Design review of the part built by this model. Coordinates are the model's own, in mm. A direction names the side the tool comes from. Give positions to 0.01 mm unless a question says otherwise; leave off trailing zeros. Order: outer loops, then holes, each group sorted by start corner. A loop starts at its lowest first (then second) coordinate and runs counter-clockwise, first axis right, second up. Notation, with made-up numbers: M 57,-8.75 L 78,-8.75 A18 ccw 78,7.25 Z; hole C 71.5,33.5 d4. An arc over 180 degrees is marked long. Answer as a JSON object with one key per item and string values.
from build123d import *

# Parameters (mm, degrees)
CHAMFER1_SIZE      = 2
CUT_EXTRUDE1_DEPTH = 5


with BuildPart() as part:
    # Sketch1 → Revolve1 (revolve)
    with BuildSketch(Plane.XY):
        Polygon((0, 0), (0, 22.5), (65, 22.5), (65, 27), (70, 27), (70, 52), (80, 52), (80, 35), (155, 35), (155, 52), (165, 52), (165, 24.5), (174, 24.5), (174, 21), (234, 21), (234, 0), align=None)
    revolve(axis=Axis((0, 0, 0), (1, 0, 0)))

    # Chamfer1
    chamfer1_edges = [part.edges().sort_by_distance(p)[0] for p in [
        (165, -24.5, 0),
        (155, -35, 0),
        (80, -35, 0),
    ]]
    chamfer(chamfer1_edges, length=CHAMFER1_SIZE)

    # Sketch2 → Cut-Extrude1 (cut)
    with BuildSketch(Plane(origin=(0, 21, 0), x_dir=(1, 0, 0), z_dir=(0, 1, 0))):
        with BuildLine():
            Line((204, 6), (204, -6))
            Line((204, -6), (184, -6))
            ThreePointArc((184, -6), (178, 0), (184, 6))
            Line((184, 6), (204, 6))
        make_face()
    cut_extrude1 = extrude(amount=-CUT_EXTRUDE1_DEPTH, mode=Mode.SUBTRACT)

    # Mirror1: Cut-Extrude1 across plane
    add(cut_extrude1.mirror(Plane(origin=(204, 16, -6), x_dir=(0, 0, 1), z_dir=(1, 0, 0))), mode=Mode.SUBTRACT)


solid = part.part
(1) We need section A-A (z = -44.5). Write out the cut boundary in (x, y).
Checked values:
{"outline": "M 70,-26.9 L 80,-26.9 L 80,26.9 L 70,26.9 Z; M 155,-26.9 L 165,-26.9 L 165,26.9 L 155,26.9 Z"}
(2) To check wall thickness, follow L1, parallel to X at y = 38, z = 28.5; L2, parallel to Z at x = 172.5, y = -1.5; L3, parallel to Y at x = 18, z = -8. State the ranges of each line that lie inside material, in increasing order. Write a range as from..to.
Checked values:
{"L1": "x = 70..80, 155..165", "L2": "z = -24.45..24.45", "L3": "y = -21.03..21.03"}
(3) Draft analysis for pull direction Z (two halves, no side actions). For faces 4 (the cylindrical face through (67.54, -5.85, -26.36)), 5 (the flat face through (174, 20, 7)), 6 (the flat face through (204, 16, 0)), state which applies: +Z half, -Z half, draft (parallel to the pull), parting line (faces both ways), or undercut.
Checked values:
{"face 4": "parting line", "face 5": "draft", "face 6": "undercut"}
(4) Insertion check: pin 1 (8 mm diameter, centred on x = 86.5, z = 34, fed in from -Y); pin 2 (4.5 mm diameter, centred on x = 212, y = 17, fed in from -Z); pin 3 (6 mm diameter, centred on y = -12, z = 26, fed in from -X). Each pin has a flat end and moves straight along its axis. Give the tip position at first contact, or say it passes through.
Checked values:
{"pin 1": "stops at y = -18.03", "pin 2": "stops at z = -14.95", "pin 3": "stops at x = 65"}
(5) We need section D-D (x = 121). Write out the cut boundary in (y, z).
Checked values:
{"outline": "C 0,0 d70"}
(6) We need section C-C (x = 55). Write out the cut boundary in (y, z), plus the area to 3 significant figures.
Checked values:
{"outline": "C 0,0 d45", "area": "1,590 mm^2"}
(7) Tool access review of faces 1 (the cylindrical face through (230, 19, 0)), 2 (the cylindrical face through (204.42, 20.03, 6.31)), 3 (the cylindrical face through (118, -28, -21)): name each direction out of +Z, -Z, +X, -X, +Y, -Y from which nothing blocks a thin tool from reaching the whole face with its end or side.
Checked values:
{"face 1": "+Y", "face 2": "+X", "face 3": "none"}
